For this review, take the finished solid that the model builds, in its own axes (mm). Face numbers are marked on the shaded views. A direction names the side the tool comes from. Coordinates: 2 decimals unless noted, no trailing zeros. Write each loop counter-clockwise with the first axis right and the second up, starting at its lowest first coordinate (ties: lowest second). Pieces come first, ordered by that corner, then holes. Notation, with made-up numbers: (-30.5, 19) -> (6.5, 19) arc R27 cw to (6.5, 55) -> close; hole circle Ø10 at (-16, -7). An arc over 180 degrees is marked (long way). Put each result on its own line as item: value. Start each with the question number.
Item 1: Insertion check: P1, Ø2, axis at x = 13.5, y = 2, coming from the -Z side; P2, Ø4.5, axis at x = 9.5, y = 0, coming from the -Z side; P3, Ø5, axis at x = 6, z = -6, coming from the -Y side. Each pin has a flat end and moves straight along its axis. Give the tip position at first contact, or say it passes through.
Item 2: Consider section A-A on y = 0. Give the boundary of the cut face in (x, z), and give its area (3 significant figures).
Item 3: For the marked faces 1, 2, 3, 4 and 5, list the 3-axis set-ups (+Z, -Z, +X, -X, +Y, -Y) from which the entire face can be reached by the end or side of a thin tool; tool diameter is ignored.
Item 4: The part is to be moulded in two halves that separate along Y. For the marked faces 6, 7, 8 and 9, say which applies: +Y half, -Y half, draft (parallel to the pull), parting line (faces both ways), or undercut.
Item 5: To check wall thickness, follow L1, parallel to Z at x = 3.5, y = -0.25; L2, parallel to Z at x = 4.5, y = -3.25; L3, parallel to X at y = 7.75, z = 3. State the ranges of each line that lie inside material, in increasing order.
Item 6: Consider section B-B on x = 5.5. Give the boundary of the cut face in (y, z), and give its area (3 significant figures).
Item 7: Consider section D-D on y = -5.5. Give the boundary of the cut face in (x, z).
Item 8: Consider section C-C on z = -1. Give the boundary of the cut face in (x, y).
Autodesk Inventor part; units mm, degrees
ref_plane "YZ Plane" through (0, 0, 0) normal (1, 0, 0) x (0, 1, 0)
ref_plane "XZ Plane" through (0, 0, 0) normal (0, 1, 0) x (-1, 0, 0)
ref_plane "XY Plane" through (0, 0, 0) normal (0, 0, 1) x (1, 0, 0)
sketch "Sketch1" plane through (0, 0, 0) normal (1, 0, 0) x (0, 1, 0)
  line L0 (0, 0) -> (3, 0) construction
  line L1 (3, 0) -> (3, -15.0663) construction
  line L2 (3, -15.0663) -> (0, -15.0663) construction
  line L3 (0, -15.0663) -> (0, 0) construction
  line L4 (0, 0) -> (-3, 0) construction
  line L5 (-3, 0) -> (-3, -15.0663) construction
  line L6 (-3, -15.0663) -> (0, -15.0663) construction
  line L7 (0, -15.0663) -> (0, 0) construction
  line L8 (3, -5.1752) -> (-2.9818, -5.1857)
  line L9 (-2.9818, -5.1857) -> (-5.9818, -0.0105)
  line L10 (-5.9818, -0.0105) -> (-3, 5.1752)
  line L11 (-3, 5.1752) -> (2.9818, 5.1857)
  line L12 (2.9818, 5.1857) -> (5.9818, 0.0105)
  line L13 (5.9818, 0.0105) -> (3, -5.1752)
  dimension "d0" = 3
  dimension "d1" = 3
extrude "Extrusion1" add sketch "Sketch1" along normal blind 3
sketch "Sketch2" plane through (0, 0, 0) normal (-1, 0, 0) x (0, 0, 1)
  point P0 (0, 0)
sketch "Sketch3" plane through (0, 0, 0) normal (-1, 0, 0) x (0, 0, 1)
  line L0 (-5.1752, 3) -> (0.0105, 5.9818)
  circle A0 centre (0, 0) radius 5.9818
extrude "Extrusion2" add sketch "Sketch3" along normal blind 2
sketch "Sketch4" plane through (3, 0, 0) normal (1, 0, 0) x (0, 0, -1)
  line L0 (0, -4.0315) -> (-3.4914, -2.0157) construction
  line L1 (-3.4914, -2.0157) -> (-3.4914, 2.0157) construction
  line L2 (-3.4914, 2.0157) -> (0, 4.0315) construction
  line L3 (0, 4.0315) -> (3.4914, 2.0157) construction
  line L4 (3.4914, 2.0157) -> (3.4914, -2.0157) construction
  line L5 (3.4914, -2.0157) -> (0, -4.0315) construction
  point P0 (0, 0)
  point P1 (0, 0)
sketch "Sketch5" plane through (3, 0, 0) normal (1, 0, 0) x (0, 0, -1)
  line L0 (0, -4.0314) -> (-3.4913, -2.0157)
  line L1 (-3.4913, -2.0157) -> (-3.4913, 2.0157)
  line L2 (-3.4913, 2.0157) -> (0, 4.0314)
  line L3 (0, 4.0314) -> (3.4913, 2.0157)
  line L4 (3.4913, 2.0157) -> (3.4913, -2.0157)
  line L5 (3.4913, -2.0157) -> (0, -4.0314)
  point P0 (0, 0)
  point P1 (0, 0)
extrude "Extrusion3" cut sketch "Sketch5" against normal blind 10
sketch "Sketch6" plane through (3, 0, 0) normal (1, 0, 0) x (0, 0, -1)
  point P0 (0, 0)
sketch "Sketch7" plane through (3, 0, 0) normal (1, 0, 0) x (0, 0, -1)
  line L0 (3.75, -6.5332) -> (-3.7829, -6.5142) construction
  line L1 (-3.7829, -6.5142) -> (-7.5329, 0.019) construction
  line L2 (-7.5329, 0.019) -> (-3.75, 6.5332) construction
  line L3 (-3.75, 6.5332) -> (3.7829, 6.5142) construction
  line L4 (3.7829, 6.5142) -> (7.5329, -0.019) construction
  line L5 (7.5329, -0.019) -> (3.75, -6.5332) construction
  line L6 (3.75, -6.5332) -> (-3.7829, -6.5142)
  line L7 (-3.7829, -6.5142) -> (-7.5329, 0.019)
  line L8 (-7.5329, 0.019) -> (-3.75, 6.5332)
  line L9 (-3.75, 6.5332) -> (3.7829, 6.5142)
  line L10 (3.7829, 6.5142) -> (7.5329, -0.019)
  line L11 (7.5329, -0.019) -> (3.75, -6.5332)
  point P0 (0, 0)
  point P1 (0, 0)
  point P2 (0, 0)
extrude "Extrusion4" add sketch "Sketch7" along normal blind 10
sketch "Sketch8" plane through (13, 0, 0) normal (1, 0, 0) x (0, 0, -1)
  circle A0 centre (0, 0) radius 8.5
  dimension "d11" = 17
extrude "Extrusion5" add sketch "Sketch8" along normal blind 2
sketch "Sketch9" plane through (-2, 0, 0) normal (-1, 0, 0) x (0, 0, 1)
  line L0 (0, -4.0314) -> (-3.4913, -2.0157)
  line L1 (-3.4913, -2.0157) -> (-3.4913, 2.0157)
  line L2 (-3.4913, 2.0157) -> (0, 4.0314)
  line L3 (0, 4.0314) -> (3.4913, 2.0157)
  line L4 (3.4913, 2.0157) -> (3.4913, -2.0157)
  line L5 (3.4913, -2.0157) -> (0, -4.0314)
  line L6 (0, -4.0314) -> (-3.4913, -2.0157)
  point P0 (0, 0)
  point P1 (0, 0)
extrude "Extrusion6" cut sketch "Sketch9" against normal blind 17.25
sketch "Sketch10" plane through (-2, 0, 0) normal (-1, 0, 0) x (0, 0, 1)
  circle A0 centre (0, 0) radius 5.9818
extrude "Extrusion7" cut sketch "Sketch10" against normal blind 5
sketch "Sketch11" plane through (3, 0, 0) normal (-1, 0, 0) x (0, 0, 1)
  line L0 (0, 6.3) -> (4.998, 6.3) construction
  line L1 (4.998, 6.3) -> (4.998, -6.3) construction
  line L2 (4.998, -6.3) -> (0, -6.3) construction
  line L3 (0, -6.3) -> (0, 6.3) construction
  line L4 (7.5329, 0.019) -> (3.75, 6.5332)
  line L5 (3.75, 6.5332) -> (7.5329, 0.019)
  line L6 (7.5329, 0.019) -> (3.7829, -6.5142)
  line L7 (3.7829, -6.5142) -> (-3.75, -6.5332)
  line L8 (-3.75, -6.5332) -> (-7.5329, -0.019)
  line L9 (-7.5329, -0.019) -> (-3.7829, 6.5142)
  line L10 (-3.7829, 6.5142) -> (3.75, 6.5332)
  line L11 (0, 6.3) -> (5.456, 3.15)
  line L12 (5.456, 3.15) -> (5.456, -3.15)
  line L13 (5.456, -3.15) -> (0, -6.3)
  line L14 (0, -6.3) -> (-5.456, -3.15)
  line L15 (-5.456, -3.15) -> (-5.456, 3.15)
  line L16 (-5.456, 3.15) -> (0, 6.3)
  point P0 (0, 0)
  point P1 (0, 0)
  point P2 (0, 0)
  dimension "d18" = 12.6
extrude "Extrusion8" cut sketch "Sketch11" against normal blind 10
properties part number "OuterLayerHub"
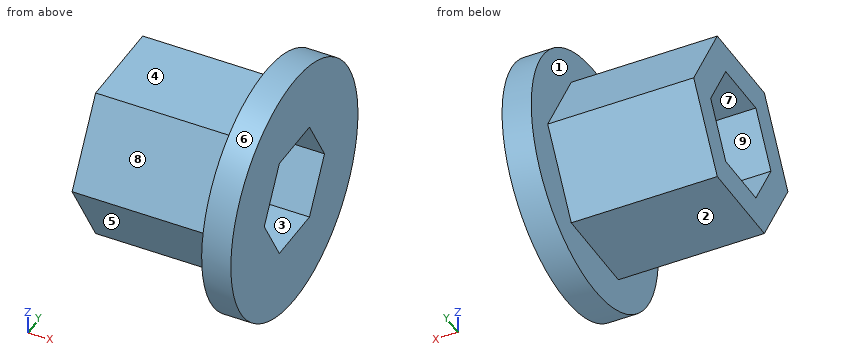
Return value:
1. P1: z = -8.44
1. P2: z = -5.46
1. P3: y = -4.28
2. outline: (3, -5.46) -> (13, -5.46) -> (13, -8.5) -> (15, -8.5) -> (15, -3.49) -> (3, -3.49) -> close; (3, 3.49) -> (15, 3.49) -> (15, 8.5) -> (13, 8.5) -> (13, 5.46) -> (3, 5.46) -> close
2. area: 59.3 mm^2
3. face 1: -X
3. face 2: -Z, -X, +Y, -Y
3. face 3: +X, -X
3. face 4: +Z, -X, +Y, -Y
3. face 5: -Z, -X, -Y
4. face 6: parting line
4. face 7: undercut
4. face 8: -Y half
4. face 9: undercut
5. L1: -5.46 to -3.49, 3.49 to 5.46
5. L2: -5.28 to -1.35, 1.35 to 5.28
5. L3: 13 to 15
6. outline: (-6.3, 0) -> (-3.15, -5.46) -> (3.15, -5.46) -> (6.3, 0) -> (3.15, 5.46) -> (-3.15, 5.46) -> close; hole (-4.03, 0) -> (-2.02, -3.49) -> (2.02, -3.49) -> (4.03, 0) -> (2.02, 3.49) -> (-2.02, 3.49) -> close
6. area: 60.9 mm^2
7. outline: (3, -1.39) -> (13, -1.39) -> (13, -6.48) -> (15, -6.48) -> (15, 6.48) -> (13, 6.48) -> (13, 1.39) -> (3, 1.39) -> close
8. outline: (3, -5.72) -> (13, -5.72) -> (13, -8.44) -> (15, -8.44) -> (15, -3.45) -> (3, -3.45) -> close; (3, 3.45) -> (15, 3.45) -> (15, 8.44) -> (13, 8.44) -> (13, 5.72) -> (3, 5.72) -> close
